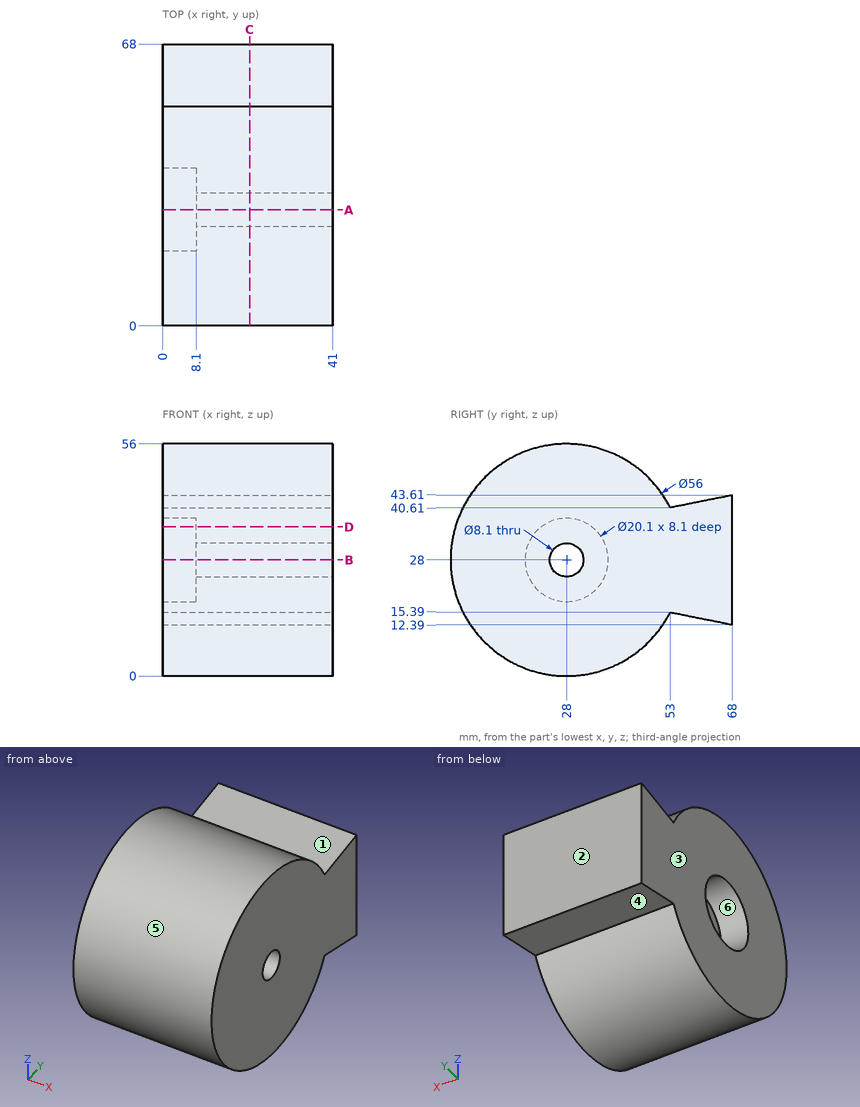
Design review of the part shown in the three views and the two pictorial views. Dimensions are in mm from the part's minimum x, y and z. A direction names the side the tool comes from. Round coordinates to 2 decimals unless told otherwise and drop trailing zeros. Write each loop counter-clockwise with the first axis right and the second up, starting at its lowest first coordinate (ties: lowest second). Pieces come first, ordered by that corner, then holes. Notation, with made-up numbers: M 60.25,83 L 110.25,83 A14 cw 110.25,96 Z; hole C 8,-8.5 d8. An arc over 180 degrees is marked long. Use a Markdown table: item, result. Add a question column.
Q1. We need section D-D, the plane z = 36. State the section outline as (x, y) points.
Q2. The part is to be moulded in two halves that separate along Y. For the marked faces 1, 2 and 3, say which applies: pulls with the +Y half, pulls with the -Y half, needs draft (parallel to the pull), parting line crosses it, or undercut.
Q3. To check wall thickness, follow line 1 (Y direction, x = 5, z = 28); line 2 (Y direction, x = 23, z = 28); line 3 (Z direction, x = 15.5, y = 28). State the ranges of each line that lie inside material, in increasing order.
Q4. We need section A-A, the plane y = 28. State the section outline as (x, z) points.
Q5. We need section C-C, the plane x = 21. State the section outline as (y, z) points, plus the area to 3 significant figures.
Q6. We need section B-B, the plane z = 28. State the section outline as (x, y) points, plus the area to 3 significant figures.
Q7. Machinability: for the marked faces 4, 5 and 6, which of the approach directions +Z, -Z, +X, -X, +Y, -Y give a long, thin tool a straight path to every point of the face, cutting with its end or side? Answer none if there is none.
Q8. Insertion check: pin 1 (10 mm diameter, centred on x = 28.5, y = 55.5, fed in from +Z) (1 decimal); pin 2 (1.5 mm diameter, centred on x = 17.5, y = 56.5, fed in from +Z); pin 3 (5 mm diameter, centred on x = 21, y = 57.5, fed in from +Z). Each pin has a flat end and moves straight along its axis. Give the tip position at first contact, or say it passes through.
Findings below:
| question | item | result |
|---|---|---|
| 1 | outline | M 0,1.17 L 41,1.17 L 41,68 L 0,68 L 0,34.08 L 8.1,34.08 L 8.1,21.92 L 0,21.92 Z |
| 2 | face 1 | undercut |
| 2 | face 2 | pulls with the +Y half |
| 2 | face 3 | needs draft |
| 3 | line 1 | y = 0 to 17.95, 38.05 to 68 |
| 3 | line 2 | y = 0 to 23.95, 32.05 to 68 |
| 3 | line 3 | z = 0 to 23.95, 32.05 to 56 |
| 4 | outline | M 0,0 L 41,0 L 41,23.95 L 8.1,23.95 L 8.1,17.95 L 0,17.95 Z; M 0,38.05 L 8.1,38.05 L 8.1,32.05 L 41,32.05 L 41,56 L 0,56 Z |
| 5 | outline | M 53,15.39 L 68,12.39 L 68,43.61 L 53,40.61 A28 ccw long Z; hole C 28,28 d8.1 |
| 5 | area | 2,780 mm² |
| 6 | outline | M 0,0 L 41,0 L 41,23.95 L 8.1,23.95 L 8.1,17.95 L 0,17.95 Z; M 0,38.05 L 8.1,38.05 L 8.1,32.05 L 41,32.05 L 41,68 L 0,68 Z |
| 6 | area | 2,360 mm² |
| 7 | face 4 | -Z, +X, -X |
| 7 | face 5 | +X, -X |
| 7 | face 6 | -X |
| 8 | pin 1 | stops at z = 44.7 |
| 8 | pin 2 | stops at z = 41.46 |
| 8 | pin 3 | stops at z = 42.01 |
